```python
from build123d import *

# Parameters (mm, degrees)
ESTRUSIONE_ESTRUSIONE1_DEPTH = 2.5
CROQUIS2_R                   = 2.05
CORTAR_EXTRUIR1_DEPTH        = 6
CUT_EXTRUDE1_REACH           = 7
SKETCH1_W                    = 4.1
SKETCH1_H                    = 30
CUT_EXTRUDE2_REACH           = 7
SKETCH2_R                    = 2.05


with BuildPart() as part:
    # Schizzo1 → Estrusione-Estrusione1 (new body, symmetric)
    with BuildSketch(Plane(origin=(0, 0, 0), x_dir=(1, 0, 0), z_dir=(0, 1, 0))):
        with BuildLine():
            Line((-25, 37.416573868), (-25, 26.25))
            Line((-25, 26.25), (25, 26.25))
            Line((25, 26.25), (25, 37.416573868))
            ThreePointArc((25, 37.416573868), (45, 0), (25, -37.416573868))
            Line((25, -37.416573868), (25, -26.25))
            Line((25, -26.25), (-25, -26.25))
            Line((-25, -26.25), (-25, -37.416573868))
            ThreePointArc((-25, -37.416573868), (-45, 0), (-25, 37.416573868))
        make_face()
    extrude(amount=ESTRUSIONE_ESTRUSIONE1_DEPTH, both=True)

    # Croquis2 → Cortar-Extruir1 (cut, through all)
    with BuildSketch(Plane(origin=(0, 2.5, 0), x_dir=(1, 0, 0), z_dir=(0, 1, 0))):
        with Locations((0, 20.25)):
            Circle(CROQUIS2_R)
        with Locations((0, -20.25)):
            Circle(CROQUIS2_R)
    extrude(amount=-CORTAR_EXTRUIR1_DEPTH, mode=Mode.SUBTRACT)

    # Sketch1 → Cut-Extrude1 (cut, up to next)
    with BuildSketch(Plane(origin=(0, 2.5, 0), x_dir=(1, 0, 0), z_dir=(0, 1, 0)), mode=Mode.PRIVATE) as cut_extrude1_sk1:
        with Locations((-20.45, 0)):
            Rectangle(SKETCH1_W, SKETCH1_H)
    cut_extrude1_tool1 = extrude(cut_extrude1_sk1.sketch, amount=-CUT_EXTRUDE1_REACH, mode=Mode.PRIVATE) & part.part
    add(cut_extrude1_tool1.solids().sort_by_distance((-20.45, 2.5, 0))[0], mode=Mode.SUBTRACT)

    # Sketch2 → Cut-Extrude2 (cut, up to next)
    with BuildSketch(Plane(origin=(0, 2.5, 0), x_dir=(1, 0, 0), z_dir=(0, 1, 0)), mode=Mode.PRIVATE) as cut_extrude2_sk1:
        with Locations((-25, 26.25)):
            Circle(SKETCH2_R)
    cut_extrude2_tool1 = extrude(cut_extrude2_sk1.sketch, amount=-CUT_EXTRUDE2_REACH, mode=Mode.PRIVATE) & part.part
    add(cut_extrude2_tool1.solids().sort_by_distance((-25, 2.5, -26.25))[0], mode=Mode.SUBTRACT)
    # Sketch2 → Cut-Extrude2 (cut, up to next)
    with BuildSketch(Plane(origin=(0, 2.5, 0), x_dir=(1, 0, 0), z_dir=(0, 1, 0)), mode=Mode.PRIVATE) as cut_extrude2_sk2:
        with Locations((-25, -26.25)):
            Circle(SKETCH2_R)
    cut_extrude2_tool2 = extrude(cut_extrude2_sk2.sketch, amount=-CUT_EXTRUDE2_REACH, mode=Mode.PRIVATE) & part.part
    add(cut_extrude2_tool2.solids().sort_by_distance((-25, 2.5, 26.25))[0], mode=Mode.SUBTRACT)
    # Sketch2 → Cut-Extrude2 (cut, up to next)
    with BuildSketch(Plane(origin=(0, 2.5, 0), x_dir=(1, 0, 0), z_dir=(0, 1, 0)), mode=Mode.PRIVATE) as cut_extrude2_sk3:
        with Locations((25, -26.25)):
            Circle(SKETCH2_R)
    cut_extrude2_tool3 = extrude(cut_extrude2_sk3.sketch, amount=-CUT_EXTRUDE2_REACH, mode=Mode.PRIVATE) & part.part
    add(cut_extrude2_tool3.solids().sort_by_distance((25, 2.5, 26.25))[0], mode=Mode.SUBTRACT)
    # Sketch2 → Cut-Extrude2 (cut, up to next)
    with BuildSketch(Plane(origin=(0, 2.5, 0), x_dir=(1, 0, 0), z_dir=(0, 1, 0)), mode=Mode.PRIVATE) as cut_extrude2_sk4:
        with Locations((25, 26.25)):
            Circle(SKETCH2_R)
    cut_extrude2_tool4 = extrude(cut_extrude2_sk4.sketch, amount=-CUT_EXTRUDE2_REACH, mode=Mode.PRIVATE) & part.part
    add(cut_extrude2_tool4.solids().sort_by_distance((25, 2.5, -26.25))[0], mode=Mode.SUBTRACT)


solid = part.part
```
Geometry check sheet. Reference: the model listing, model coordinates, mm. A direction names the side the tool comes from. Coordinates: 2 decimals unless noted, no trailing zeros. Order: outer loops, then holes, each group sorted by start corner. A loop starts at its lowest first (then second) coordinate and runs counter-clockwise, first axis right, second up. Notation, with made-up numbers: M 76,44 L 110,44 A18 ccw 110,57 Z; hole C 15,-6.5 d8. An arc over 180 degrees is marked long. One line per question, with ' | ' between items. Start each with the question number.
Item 1: Cross-section at A-A on x = 0. Enter the section's corners in (y, z), then the cut area to 4 significant figures.
Item 2: Draft check along X on faces 4 (the cylindrical face through (26.4, 0.04, -24.75)), 5 (the flat face through (1, 2.5, -1)), 6 (the cylindrical face through (44.996, 0.035, -0.618)). Enter one of: pulls with the +X half, pulls with the -X half, needs draft (parallel to the pull), parting line crosses it, or undercut.
Item 3: Cross-section at C-C on z = 20.25. Enter the section's corners in (x, y), then the cut area to 3 significant figures.
Item 4: Set-up check for faces 1 (the flat face through (0, 0, -26.25)), 2 (the flat face through (25, 0, 33)), 3 (the flat face through (-22.5, 0, 0)): record each of +Z, -Z, +X, -X, +Y, -Y from which the full face is reachable in a straight line by a thin tool's end or side.
Item 5: Cross-section at D-D on x = 18. Enter the section's corners in (y, z), then the cut area to 4 significant figures.
Item 6: Material ranges on L1, parallel to Z at x = 0, y = -1.2; L2, parallel to Z at x = -16.5, y = 1.9, recorded low to high. Write a range as [from, to].
Item 7: Gauge pin test, flat ends, axial feed: pin 1 (1.5 mm diameter, centred on y = 1, z = 30.5, fed in from -X); pin 2 (1.2 mm diameter, centred on x = -21.5, y = -1, fed in from +Z); pin 3 (2.5 mm diameter, centred on y = 0.5, z = -34.5, fed in from +X). Record the tip position at first contact, or that the pin passes through.
Item 8: Cross-section at B-B on y = 0.6. Enter the section's corners in (x, z), then the cut area to 3 significant figures.
Findings:
1) outline: M -2.5,-26.25 L 2.5,-26.25 L 2.5,-22.3 L -2.5,-22.3 Z; M -2.5,-18.2 L 2.5,-18.2 L 2.5,18.2 L -2.5,18.2 Z; M -2.5,22.3 L 2.5,22.3 L 2.5,26.25 L -2.5,26.25 Z | area: 221.5 mm²
2) face 4: undercut | face 5: needs draft | face 6: pulls with the +X half
3) outline: M -40.19,-2.5 L -2.05,-2.5 L -2.05,2.5 L -40.19,2.5 Z; M 2.05,-2.5 L 40.19,-2.5 L 40.19,2.5 L 2.05,2.5 Z | area: 381 mm²
4) face 1: -Z, +Y, -Y | face 2: +Z, +Y, -Y | face 3: +Y, -Y
5) outline: M -2.5,-26.25 L 2.5,-26.25 L 2.5,26.25 L -2.5,26.25 Z | area: 262.5 mm²
6) L1: z = [-26.25, -22.3], [-18.2, 18.2], [22.3, 26.25] | L2: z = [-26.25, 26.25]
7) pin 1: stops at x = -33.76 | pin 2: stops at z = 26.25 | pin 3: stops at x = 30.32
8) outline: M -25,-37.42 L -25,-28.3 A2.05 cw long -22.95,-26.25 L 22.95,-26.25 A2.05 cw long 25,-28.3 L 25,-37.42 A45 ccw 25,37.42 L 25,28.3 A2.05 cw long 22.95,26.25 L -22.95,26.25 A2.05 cw long -25,28.3 L -25,37.42 A45 ccw Z; hole M -22.5,-15 L -18.4,-15 L -18.4,15 L -22.5,15 Z; hole C 0,-20.25 d4.1; hole C 0,20.25 d4.1 | area: 4,540 mm²
